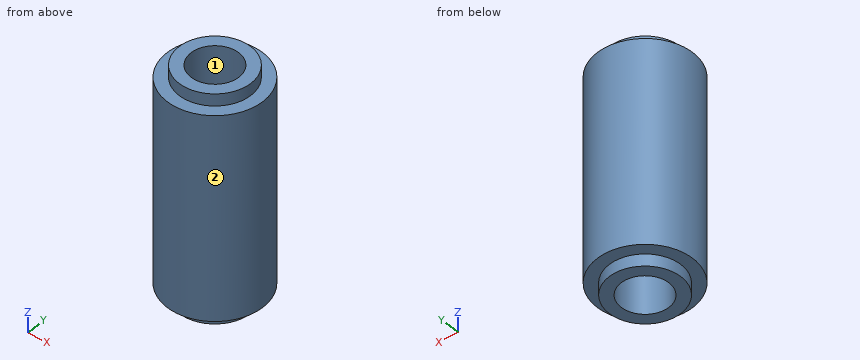
Autodesk Inventor part; units mm, degrees
ref_plane "YZ Plane" through (0, 0, 0) normal (1, 0, 0) x (0, 1, 0)
ref_plane "XZ Plane" through (0, 0, 0) normal (0, 1, 0) x (-1, 0, 0)
ref_plane "XY Plane" through (0, 0, 0) normal (0, 0, 1) x (1, 0, 0)
sketch "Sketch1" plane through (0, 0, 0) normal (0, 0, 1) x (1, 0, 0)
  circle A0 centre (0, 0) radius 6.35
  circle A1 centre (0, 0) radius 3.175
  dimension "d0" = 12.7
  dimension "d13" = 3.175
extrude "Base" add sketch "Sketch1" along normal mid plane 30.1625
sketch "Sketch4" plane through (0, 0, 15.0812) normal (0, 0, 1) x (1, 0, 0)
  circle A0 centre (0, 0) radius 6.35
  circle A1 centre (0, 0) radius 4.7625
  dimension "d16" = 9.525
extrude "Extrusion4" cut sketch "Sketch4" against normal blind 1.5875
mirror "Mirror2" about plane through (0, 0, 0) normal (0, 0, 1) of "Extrusion4"
properties part number "gearbox_standoff" material "Aluminum-6061"
Part model, mm, in its own coordinate system. Face numbers are marked on the shaded views. Give positions to 0.01 mm unless a question says otherwise; leave off trailing zeros. Write each loop counter-clockwise with the first axis right and the second up, starting at its lowest first coordinate (ties: lowest second). Pieces come first, ordered by that corner, then holes. Notation, with made-up numbers: (23, 0.5) -> (68, 0.5) arc R14 ccw to (68, 27.5) -> close; hole circle Ø8 at (5, -30.75). An arc over 180 degrees is marked (long way). Put each result on its own line as item: value. Start each with the question number.
Item 1: Pull direction X, two halves, no side cores. Call the marked faces 1 and 2: pulls with the +X half, pulls with the -X half, needs draft (parallel to the pull), parting line crosses it, or undercut.
Item 2: Pin check, flat tips, straight feed: pin 1 Ø1 at (y, z) = (4.5, -0.5) entering from +X; pin 2 Ø1 at (y, z) = (-2, 2) entering from +X; pin 3 Ø3 at (x, z) = (-5, -11.5) entering from +Y. Stop position of each tip, or through.
Item 3: Wall check: L1, parallel to Y at x = 0, z = 6 (3 decimals); L2, parallel to Z at x = -0.25, y = 5.5; L3, parallel to Y at x = 1.75, z = 13. Give the ranges that are in metal, low to high. Write a range as [from, to].
Item 4: Cut at C-C (z = -2.5). List the corners of the cut face in (x, y) (3 decimals).
Item 5: Cut at D-D (y = -4). List the corners of the cut face in (x, z).
Answer list:
1. face 1: undercut
1. face 2: parting line crosses it
2. pin 1: stops at x = 4.93
2. pin 2: stops at x = 6.17
2. pin 3: stops at y = 5.3
3. L1: y = [-6.35, -3.175], [3.175, 6.35]
3. L2: z = [-13.49, 13.49]
3. L3: y = [-6.1, -2.65], [2.65, 6.1]
4. outline: circle Ø12.7 at (0, 0); hole circle Ø6.35 at (0, 0)
5. outline: (-4.93, -13.49) -> (-2.58, -13.49) -> (-2.58, -15.08) -> (2.58, -15.08) -> (2.58, -13.49) -> (4.93, -13.49) -> (4.93, 13.49) -> (2.58, 13.49) -> (2.58, 15.08) -> (-2.58, 15.08) -> (-2.58, 13.49) -> (-4.93, 13.49) -> close
